Drawing for the job (mm, zero at the part's lowest x, y, z). Give positions to 0.01 mm unless a question says otherwise; leave off trailing zeros. Order: outer loops, then holes, each group sorted by start corner. A loop starts at its lowest first (then second) coordinate and runs counter-clockwise, first axis right, second up. Notation, with made-up numbers: M 76,32 L 127,32 A29 cw 127,57 Z; hole C 63,78.5 d11. An arc over 180 degrees is marked long. Answer as a JSON object with one key per item and string values.
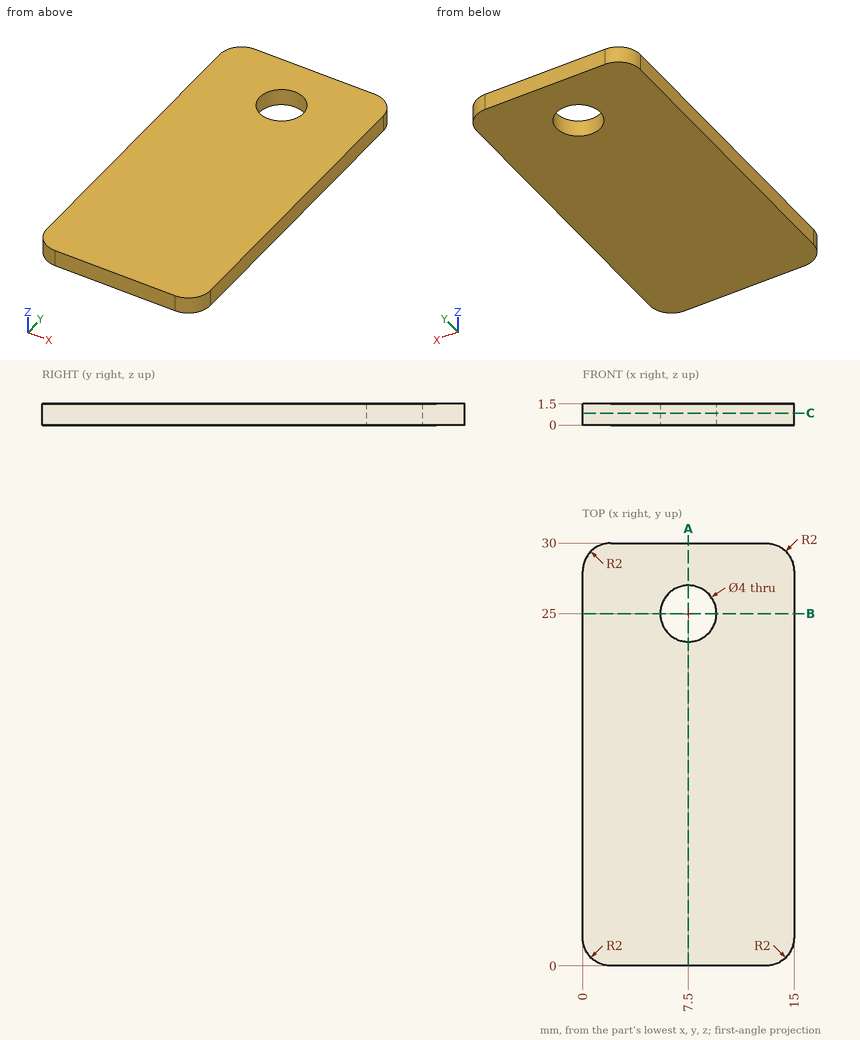
1. Cut at C-C on z = 0.85. Give the cut face in (x, y), plus the area to 3 significant figures.
Worked answers:
{"outline": "M 0,2 A2 ccw 2,0 L 13,0 A2 ccw 15,2 L 15,28 A2 ccw 13,30 L 2,30 A2 ccw 0,28 Z; hole C 7.5,25 d4", "area": "434 mm^2"}
2. Cut at A-A on x = 7.5. Give the cut face in (y, z), plus the area to 3 significant figures.
Worked answers:
{"outline": "M 0,0 L 23,0 L 23,1.5 L 0,1.5 Z; M 27,0 L 30,0 L 30,1.5 L 27,1.5 Z", "area": "39.0 mm^2"}
3. Probe line 1 along Y through (x, z) = (7.5, 0.3); line 2 along Y through (x, z) = (6, 0.75); line 3 along X through (y, z) = (25.75, 1.25). List the from-to ranges inside material, lowest first.
Worked answers:
{"line 1": "y = 0 to 23, 27 to 30", "line 2": "y = 0 to 23.68, 26.32 to 30", "line 3": "x = 0 to 5.65, 9.35 to 15"}
4. Cut at B-B on y = 25. Give the cut face in (x, z), plus the area to 3 significant figures.
Worked answers:
{"outline": "M 0,0 L 5.5,0 L 5.5,1.5 L 0,1.5 Z; M 9.5,0 L 15,0 L 15,1.5 L 9.5,1.5 Z", "area": "16.5 mm^2"}
